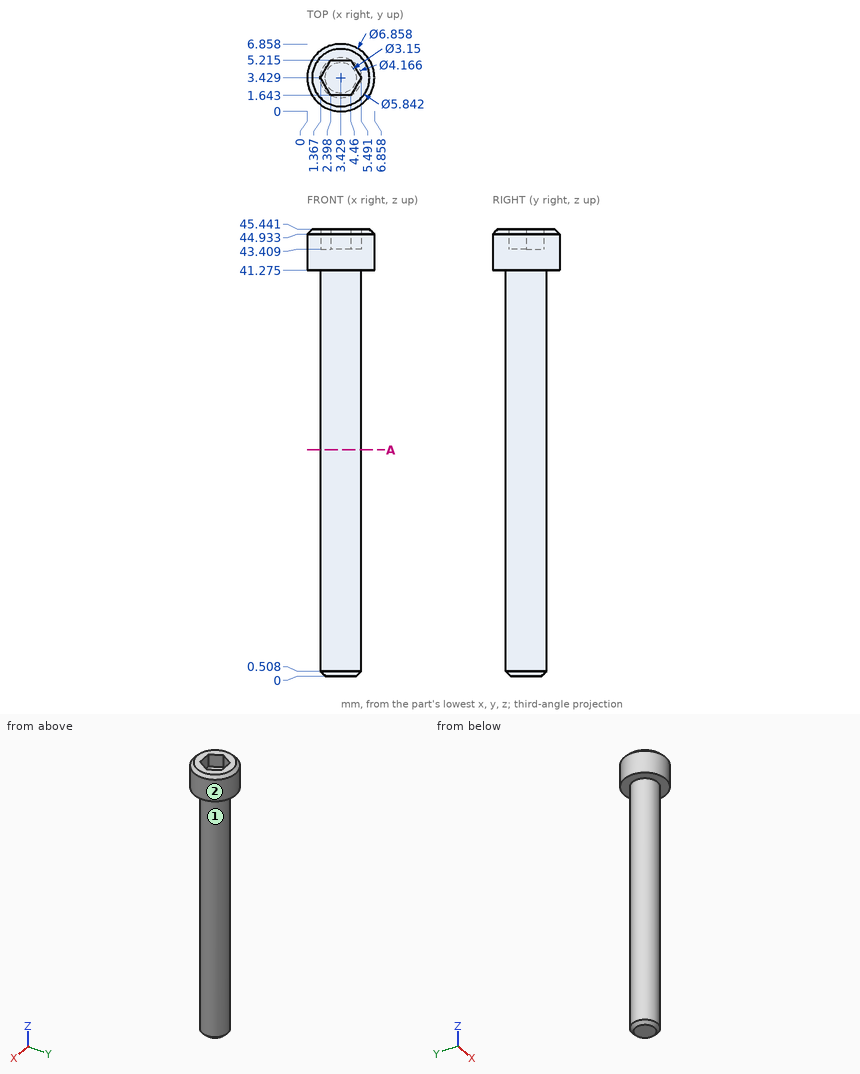
Could you check a few things on this drawing? It's one solid part, dimensions in mm from its lowest x, y, z. A direction names the side the tool comes from. Give positions to 0.01 mm unless a question says otherwise; leave off trailing zeros. Order: outer loops, then holes, each group sorted by start corner. A loop starts at its lowest first (then second) coordinate and runs counter-clockwise, first axis right, second up. Notation, with made-up numbers: (-9.75, 34) -> (5.25, 34) arc R17 cw to (5.25, 41) -> close; hole circle Ø3 at (59, 41.25). An arc over 180 degrees is marked (long way). Answer in a Markdown table with one row per item. Add a question column.
Item 1: Imagine slicing it at A-A (z = 23). List the corners of the cut face in (x, y) for me (1 decimal).
Item 2: For the marked faces 1 and 2, which set-ups out of +Z, -Z, +X, -X, +Y, -Y let a thin tool reach every point of the face, with its end or its side?
Item 3: I'm going to push flat-ended pins straight in: P1, Ø4, axis at y = 4, z = 16, coming from the +X side; P2, Ø3, axis at x = 1.5, z = 37, coming from the +Y side; P3, Ø1.5, axis at y = 2, z = 40, coming from the +X side. Where does each tip first touch, or does it pass through?
Item 4: Please list where these lines run through material, in increasing order: probe 1 along X at (y, z) = (3.5, 28.5); probe 2 along Z at (x, y) = (4.5, 2.5); probe 3 along Y at (x, z) = (4.5, 17.5) (1 decimal).
Result:
| question | item | result |
|---|---|---|
| 1 | outline | circle Ø4.2 at (3.4, 3.4) |
| 2 | face 1 | -Z |
| 2 | face 2 | +Z, -Z |
| 3 | P1 | x = 5.51 |
| 3 | P2 | y = 5.47 |
| 3 | P3 | x = 5.4 |
| 4 | probe 1 | 1.35 to 5.51 |
| 4 | probe 2 | 0 to 43.41 |
| 4 | probe 3 | 1.6 to 5.2 |
